from build123d import *

# Parameters (mm, degrees)
SKETCH1_R           = 2.702962803
SKETCH1_R_2         = 2.510598202
BOSS_EXTRUDE1_DEPTH = 30


with BuildPart() as part:
    # Sketch1 → Boss-Extrude1 (new body)
    with BuildSketch(Plane.XY):
        with BuildLine():
            Line((-42.5, -8.80249494), (-42.5, -18.80249494))
            ThreePointArc((-42.5, -18.80249494), (0, -36.80249494), (42.5, -18.80249494))
            Line((42.5, -18.80249494), (42.5, -8.80249494))
            ThreePointArc((42.5, -8.80249494), (48.855409625, -11.804679997), (55, -15.217648755))
            Line((55, -15.217648755), (49.831703302, -20.194115642))
            Line((49.831703302, -20.194115642), (43.936451121, -20.194115642))
            ThreePointArc((43.936451121, -20.194115642), (0, -38.80249494), (-43.936451121, -20.194115642))
            Line((-43.936451121, -20.194115642), (-49.831703302, -20.194115642))
            Line((-49.831703302, -20.194115642), (-55, -15.217648755))
            ThreePointArc((-55, -15.217648755), (-48.855409625, -11.804679997), (-42.5, -8.80249494))
        make_face()
        with Locations((-48, -15.80249494)):
            Circle(SKETCH1_R, mode=Mode.SUBTRACT)
        with Locations((48, -15.80249494)):
            Circle(SKETCH1_R_2, mode=Mode.SUBTRACT)
    extrude(amount=BOSS_EXTRUDE1_DEPTH)


solid = part.part
Could you check a few things on this model? Use its own coordinates, in mm. A direction names the side the tool comes from. Coordinates: 2 decimals unless noted, no trailing zeros. Loops run counter-clockwise (first coordinate to the right, second up) from the corner with the lowest first, then second, coordinate; pieces in that order, holes last.
1. For P1, Ø6, axis at y = -22.5, z = 7, coming from the -X side; P2, Ø4.5, axis at x = -46.5, z = 9, coming from the -Y side; P3, Ø11, axis at y = -14, z = 18, coming from the +X side, each with a flat end and sliding along its axis, tell me the tip position at first contact or that it passes through.
2. Imagine slicing it at B-B (y = -23). Please give me the cut outline in (x, z).
3. We'd pull the mould along Y, two halves only. Please class faces 6 (the face through (-52.38, -17.74, 14.79)), 7 (the face through (42.5, -14, 15)), 8 (the face through (-45.42, -14.99, 14.79)): released by +Y, released by -Y, zero draft, split by the parting line, or undercut.
4. For faces 1 (the face through (-47, -20.194, 15)), 2 (the face through (47, -20.194, 15)), 3 (the face through (0.7, -38.8, 14.8)), 4 (the face through (-42.5, -14, 15)), 5 (the face through (48.77, -11.76, 14.79)), which set-ups out of +Z, -Z, +X, -X, +Y, -Y let a thin tool reach every point of the face, with its end or its side?
5. Imagine slicing it at D-D (x = -28). Please give me the cut outline in (y, z), and give its area (3 significant figures).
6. Imagine slicing it at A-A (x = 48). Please give me the cut outline in (y, z), and give its area (3 significant figures).
7. I need wall thicknesses on L1, parallel to X at y = -17, z = 28.25; L2, parallel to X at y = -15, z = 11; L3, parallel to Y at x = 48, z = 20.75. Which ranges of each line are inside material? Lowest first, please.
8. Imagine slicing it at C-C (z = 14.5). Please give me the cut outline in (x, y).
Computed values:
1. P1: stops at x = -50.55
1. P2: stops at y = -20.19
1. P3: stops at x = 55
2. outline: (-41.03, 0) - (-37.99, 0) - (-37.99, 30) - (-41.03, 30) - close; (37.99, 0) - (41.03, 0) - (41.03, 30) - (37.99, 30) - close
3. face 6: released by -Y
3. face 7: zero draft
3. face 8: undercut
4. face 1: +Z, -Z, -X, -Y
4. face 2: +Z, -Z, +X, -Y
4. face 3: +Z, -Z, -Y
4. face 4: +Z, -Z, +Y
4. face 5: +Z, -Z, +X, +Y
5. outline: (-32.02, 0) - (-29.76, 0) - (-29.76, 30) - (-32.02, 30) - close
5. area: 67.8 mm2
6. outline: (-20.19, 0) - (-18.31, 0) - (-18.31, 30) - (-20.19, 30) - close; (-13.29, 0) - (-11.37, 0) - (-11.37, 30) - (-13.29, 30) - close
6. area: 114 mm2
7. L1: x = -53.15 to -50.42, -45.58 to -42.5, 42.5 to 45.79, 50.21 to 53.15
7. L2: x = -54.64 to -50.58, -45.42 to -42.5, 42.5 to 45.62, 50.38 to 54.64
7. L3: y = -20.19 to -18.31, -13.29 to -11.37
8. outline: (-55, -15.22) - (-49.83, -20.19) - (-43.94, -20.19) arc R61.17 ccw to (43.94, -20.19) - (49.83, -20.19) - (55, -15.22) arc R107 ccw to (42.5, -8.8) - (42.5, -18.8) arc R59.17 cw to (-42.5, -18.8) - (-42.5, -8.8) arc R107 ccw to start; hole circle Ø5.41 at (-48, -15.8); hole circle Ø5.02 at (48, -15.8)
